Can you work these out from the model? Positions are in its coordinate system, mm. A direction names the side the tool comes from. Give positions to 0.01 mm unless a question says otherwise; leave off trailing zeros. Loops run counter-clockwise (first coordinate to the right, second up) from the corner with the lowest first, then second, coordinate; pieces in that order, holes last. Notation, with made-up numbers: (8, 1.5) - (54, 1.5) arc R22 ccw to (54, 16.5) - close; hole circle Ø4 at (8.25, 85.5). An arc over 180 degrees is marked (long way). Answer as a JSON object with one key per item and string values. Group by question number.
Item 1: Suppose I cut it at B-B on x = 27. Write out the boundary of the cut face in (y, z), and give its area (4 significant figures).
Item 2: Please list where these lines run through material, in increasing order: L1, parallel to Z at x = 33, y = -8.5; L2, parallel to Y at x = 25.5, z = 14.
Item 3: Suppose I cut it at C-C on z = 40. Write out the boundary of the cut face in (x, y).
Item 4: Will this pin go through, and if not, where does the flat tip stop? pin 1 (6 mm diameter, centred on x = -11, z = 14.5, fed in from -Y).
Item 5: Thinking about a two-plate mould opening in Z: for faces 1 (the flat face through (-1, 1, -82.5)), 2 (the flat face through (-1, -1, 82.5)), 3 (the flat face through (-1, -1, 81)), which applies, pulls with the +Z half, pulls with the -Z half, needs draft (parallel to the pull), parting line crosses it, or undercut?
Item 6: Which directions (+Z, -Z, +X, -X, +Y, -Y) give clear straight access to the entire face, cutting with the end or side of a thin tool? Please do faces 4 (the flat face through (-1, 44.25, 1)), 5 (the flat face through (-1, 45.75, 1)).
Item 7: Suppose I cut it at A-A on y = 37. Write out the boundary of the cut face in (x, z).
Autodesk Inventor part; units mm, degrees
ref_plane "YZ Plane" through (0, 0, 0) normal (1, 0, 0) x (0, 1, 0)
ref_plane "XZ Plane" through (0, 0, 0) normal (0, 1, 0) x (-1, 0, 0)
ref_plane "XY Plane" through (0, 0, 0) normal (0, 0, 1) x (1, 0, 0)
sketch "Skizze1" plane through (0, 0, 0) normal (1, 0, 0) x (0, 1, 0)
  line L0 (-45.75, 82.5) -> (45.75, 82.5)
  line L1 (45.75, 82.5) -> (45.75, -82.5)
  line L2 (45.75, -82.5) -> (-45.75, -82.5)
  line L3 (-45.75, 81) -> (44.25, 81)
  line L4 (44.25, 81) -> (44.25, -81)
  line L5 (44.25, -81) -> (-45.75, -81)
  line L6 (-45.75, -82.5) -> (-45.75, -81)
  line L7 (-45.75, 81) -> (-45.75, 82.5)
  point P0 (0, 0)
  point P1 (0, 82.5)
  point P2 (45.75, 0)
  dimension "d0" = 1.5
  dimension "d1" = 1.5
  dimension "d2" = 1.5
  dimension "d3" = 90
  dimension "d4" = 165
extrude "Extrusion1" add sketch "Skizze1" along normal mid plane 91
sketch "Skizze2" plane through (-45.5, 45.75, 82.5) normal (0, 1, 0) x (1, 0, 0)
  line L0 (64, 105) -> (27, 105)
  line L1 (27, 105) -> (27, 135)
  line L2 (27, 135) -> (64, 135)
  line L3 (64, 135) -> (64, 105)
  line L4 (91, 165) -> (0, 165)
  line L5 (91, 165) -> (91, 0)
  line L6 (0, 0) -> (0, 165)
  point P0 (45.5, 82.5)
  dimension "d7" = 30
  dimension "d8" = 30
  dimension "d9" = 27
  dimension "d10" = 27
extrude "Extrusion2" cut sketch "Skizze2" against normal through all
properties part number "Platinenhalter"
Worked out:
{
 "1": {"outline": "(-45.75, -82.5) - (45.75, -82.5) - (45.75, 82.5) - (-45.75, 82.5) - (-45.75, 81) - (44.25, 81) - (44.25, -81) - (-45.75, -81) - close", "area": "517.5 mm2"},
 "2": {"L1": "z = -82.5 to -81, 81 to 82.5", "L2": "y = 44.25 to 45.75"},
 "3": {"outline": "(-45.5, 44.25) - (45.5, 44.25) - (45.5, 45.75) - (-45.5, 45.75) - close"},
 "4": {"pin 1": "stops at y = 44.25"},
 "5": {"face 1": "pulls with the -Z half", "face 2": "pulls with the +Z half", "face 3": "undercut"},
 "6": {"face 4": "+X, -X, -Y", "face 5": "+Z, -Z, +X, -X, +Y"},
 "7": {"outline": "(-45.5, -82.5) - (45.5, -82.5) - (45.5, -81) - (-45.5, -81) - close; (-45.5, 81) - (45.5, 81) - (45.5, 82.5) - (-45.5, 82.5) - close"}
}
